Build history of the part. All positions in model axes, mm. Face numbers are marked on the shaded views. A direction names the side the tool comes from. Round coordinates to 2 decimals unless told otherwise and drop trailing zeros. Order: outer loops, then holes, each group sorted by start corner. A loop starts at its lowest first (then second) coordinate and runs counter-clockwise, first axis right, second up. Notation, with made-up numbers: M 3,86 L 35,86 A21 ccw 35,105 Z; hole C -24.75,70.5 d4. An arc over 180 degrees is marked long. One line per question, with ' | ' between items. Start each with the question number.
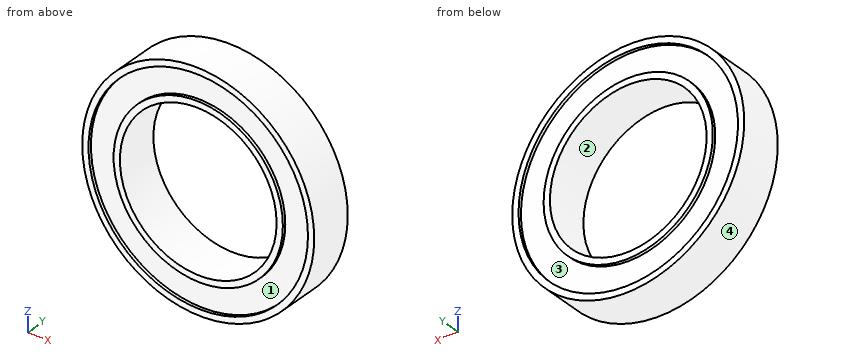
from build123d import *

# Parameters (mm, degrees)
SKETCH_1_R             = 18.5
SKETCH_1_R_2           = 17.5
EXTRUDE_1_DEPTH        = 3.5
EXTRUDE_1_DEPTH_BACK   = 3.5
SKETCH_1_R_3           = 13.5
SKETCH_1_R_4           = 12.5
EXTRUDE_1_2_DEPTH      = 3.5
EXTRUDE_1_2_DEPTH_BACK = 3.5
SKETCH_2_R             = 17.5
SKETCH_2_R_2           = 13.5
EXTRUDE_2_DEPTH        = 3
EXTRUDE_2_DEPTH_BACK   = 3


with BuildPart() as part:
    # Sketch 1 → Extrude 1 (new body, two sides)
    with BuildSketch(Plane(origin=(0, 0, 0), x_dir=(1, 0, 0), z_dir=(0, 1, 0))) as extrude_1_sk:
        Circle(SKETCH_1_R)
        Circle(SKETCH_1_R_2, mode=Mode.SUBTRACT)
    extrude(amount=EXTRUDE_1_DEPTH)
    extrude(extrude_1_sk.sketch, amount=-EXTRUDE_1_DEPTH_BACK)



with BuildPart() as body_2:
    # Sketch 1 → Extrude 1 2 (new body, two sides)
    with BuildSketch(Plane(origin=(0, 0, 0), x_dir=(1, 0, 0), z_dir=(0, 1, 0))) as extrude_1_2_sk:
        Circle(SKETCH_1_R_3)
        Circle(SKETCH_1_R_4, mode=Mode.SUBTRACT)
    extrude(amount=EXTRUDE_1_2_DEPTH)
    extrude(extrude_1_2_sk.sketch, amount=-EXTRUDE_1_2_DEPTH_BACK)


with BuildPart() as part_1:
    add(part.part)

    add(body_2.part)  # Extrude 2 merges body 2
    # Sketch 2 → Extrude 2 (add, two sides)
    with BuildSketch(Plane(origin=(0, 0, 0), x_dir=(1, 0, 0), z_dir=(0, 1, 0))) as extrude_2_sk:
        Circle(SKETCH_2_R)
        Circle(SKETCH_2_R_2, mode=Mode.SUBTRACT)
    extrude(amount=EXTRUDE_2_DEPTH)
    extrude(extrude_2_sk.sketch, amount=-EXTRUDE_2_DEPTH_BACK)


solid = part_1.part
Item 1: Cut at A-A on x = 0. Write the cut outline in (y, z).
Item 2: Cut at C-C on y = -2. Write the cut outline in (x, z), then the cut area to 3 significant figures.
Item 3: Two-plate mould, pull along Z, no slides. Class the marked faces 3 and 4: +Z half, -Z half, draft (parallel to the pull), parting line (faces both ways), or undercut.
Item 4: Flat gauge pins, fed straight in: pin 1 (4 mm diameter, centred on y = -0.5, z = 13, fed in from +X); pin 2 (1 mm diameter, centred on x = 5, y = 2, fed in from -Z); pin 3 (1.5 mm diameter, centred on x = -9, y = 0.5, fed in from +Z); pin 4 (1 mm diameter, centred on x = -5, z = -10.5, fed in from +Y). Where does each tip first touch, or does it go through?
Item 5: Wall check: line 1 along Z through (x, y) = (0, 3.25); line 2 along X through (y, z) = (2.25, 0). Give the ranges that are in metal, low to high. Write a range as [from, to].
Item 6: Cut at B-B on z = 0. Write the cut outline in (x, y), then the cut area to 3 significant figures.
Item 7: Tool access for the marked faces 1 and 2: list every direction of +Z, -Z, +X, -X, +Y, -Y with a clear straight run to the whole face (end or side of a thin tool).
Item 8: Cut at D-D on z = 15. Write the cut outline in (x, y).
Results found:
1) outline: M -3.5,-18.5 L 3.5,-18.5 L 3.5,-17.5 L 3,-17.5 L 3,-13.5 L 3.5,-13.5 L 3.5,-12.5 L -3.5,-12.5 L -3.5,-13.5 L -3,-13.5 L -3,-17.5 L -3.5,-17.5 Z; M -3.5,12.5 L 3.5,12.5 L 3.5,13.5 L 3,13.5 L 3,17.5 L 3.5,17.5 L 3.5,18.5 L -3.5,18.5 L -3.5,17.5 L -3,17.5 L -3,13.5 L -3.5,13.5 Z
2) outline: C 0,0 d37; hole C 0,0 d25 | area: 584 mm^2
3) face 3: undercut | face 4: parting line
4) pin 1: stops at x = 14.87 | pin 2: stops at z = -17.94 | pin 3: stops at z = 16.56 | pin 4: passes through
5) line 1: z = [-18.5, -17.5], [-13.5, -12.5], [12.5, 13.5], [17.5, 18.5] | line 2: x = [-18.5, -12.5], [12.5, 18.5]
6) outline: M -18.5,-3.5 L -17.5,-3.5 L -17.5,-3 L -13.5,-3 L -13.5,-3.5 L -12.5,-3.5 L -12.5,3.5 L -13.5,3.5 L -13.5,3 L -17.5,3 L -17.5,3.5 L -18.5,3.5 Z; M 12.5,-3.5 L 13.5,-3.5 L 13.5,-3 L 17.5,-3 L 17.5,-3.5 L 18.5,-3.5 L 18.5,3.5 L 17.5,3.5 L 17.5,3 L 13.5,3 L 13.5,3.5 L 12.5,3.5 Z | area: 76.0 mm^2
7) face 1: -Y | face 2: +Y, -Y
8) outline: M -10.83,-3.5 L -9.01,-3.5 L -9.01,-3 L 9.01,-3 L 9.01,-3.5 L 10.83,-3.5 L 10.83,3.5 L 9.01,3.5 L 9.01,3 L -9.01,3 L -9.01,3.5 L -10.83,3.5 Z
